Input: part model. Units: mm. Frame: model coordinates. A direction names the side the tool comes from. Coordinates: 2 decimals unless noted, no trailing zeros. Order: outer loops, then holes, each group sorted by start corner. A loop starts at its lowest first (then second) coordinate and runs counter-clockwise, first axis right, second up. Notation, with made-up numbers: (-35, 35) -> (-12, 35) arc R26 cw to (-12, 69) -> close; hole circle Ø9 at (61, 1.5). An arc over 180 degrees is marked (long way). Use one line per item in the form item = value. Start each with the question number.
1) Section query C-C on z = 0. Output: boundary loops of the cut face in (x, y) (3 decimals), then the cut area to 3 significant figures.
2) Section query B-B on y = -2.25. Output: boundary loops of the cut face in (x, z).
3) Section query D-D on z = -5.5. Output: boundary loops of the cut face in (x, y) (3 decimals), then the cut area to 3 significant figures.
4) Draft query along Y for faces 1 (the cylindrical face through (-6.97, -7.02, 0.16)), 2 (the flat face through (-3, -12.7, 3)), 3 (the cylindrical face through (-10.279, 8.343, 0.078)), 4 (the flat face through (-12.7, -3, 3)). Return one class per face: pulls with the +Y half, pulls with the -Y half, needs draft (parallel to the pull), parting line crosses it, or undercut.
5) Pin query (flat end, axial travel): pin 1 (6.5 mm diameter, centred on x = 4, z = -4.5, fed in from +Y); pin 2 (2 mm diameter, centred on x = -9, z = -7, fed in from +Y); pin 3 (11.5 mm diameter, centred on x = 0, z = 0, fed in from +Y). Return the tip coordinate at first contact, or that it passes through.
6) Ray query, line 1 along Z through (x, y) = (0, -11.2); line 2 along Y through (x, z) = (-2.25, 3); line 3 along Y through (x, z) = (-9.5, -0.25). Return the intervals inside material, ascending.
7) Access query for faces 5 (the cylindrical face through (-10.279, -3.568, -0.078)), 6 (the cylindrical face through (-3.565, -10.279, -0.157)), 7 (the flat face through (4, -7.925, 0)). Directions: +Z, -Z, +X, -X, +Y, -Y. A direction counts if a zero-diameter tool reaches every point of the face in a straight line with its end or side. Return the directions, or none.
8) Section query A-A on x = 0. Output: boundary loops of the cut face in (y, z).
from build123d import *

# Parameters (mm, degrees)
BOSS_EXTRUDE1_DEPTH      = 11.1125
BOSS_EXTRUDE1_DEPTH_BACK = 11.1125
CUT_EXTRUDE1_DEPTH       = 21.6248
CUT_EXTRUDE1_DEPTH_BACK  = 5.7752
SKETCH6_R                = 3.5687
CUT_EXTRUDE2_DEPTH       = 5.7752


with BuildPart() as part:
    # Sketch4 → Boss-Extrude1 (new body, two sides)
    with BuildSketch(Plane.XY) as boss_extrude1_sk:
        with BuildLine():
            Line((-12.7, 12.7), (-12.7, -12.7))
            Line((-12.7, -12.7), (12.7, -12.7))
            ThreePointArc((12.7, -12.7), (11.301376302, -9.323423698), (7.9248, -7.9248))
            Line((7.9248, -7.9248), (-4.7498, -7.9248))
            ThreePointArc((-4.7498, -7.9248), (-6.99486403, -6.99486403), (-7.9248, -4.7498))
            Line((-7.9248, -4.7498), (-7.9248, 7.9248))
            ThreePointArc((-7.9248, 7.9248), (-9.323423698, 11.301376302), (-12.7, 12.7))
        make_face()
    extrude(amount=BOSS_EXTRUDE1_DEPTH)
    extrude(boss_extrude1_sk.sketch, amount=-BOSS_EXTRUDE1_DEPTH_BACK)

    # Sketch5 → Cut-Extrude1 (cut, two sides)
    with BuildSketch(Plane(origin=(-7.9248, 0, 0), x_dir=(0, 0, -1), z_dir=(1, 0, 0))) as cut_extrude1_sk:
        with BuildLine():
            Line((3.5687, 4.7752), (3.5687, 0))
            ThreePointArc((3.5687, 0), (0, -3.5687), (-3.5687, 0))
            Line((-3.5687, 0), (-3.5687, 4.7752))
            ThreePointArc((-3.5687, 4.7752), (0, 8.3439), (3.5687, 4.7752))
        make_face()
    extrude(amount=CUT_EXTRUDE1_DEPTH, mode=Mode.SUBTRACT)
    extrude(cut_extrude1_sk.sketch, amount=-CUT_EXTRUDE1_DEPTH_BACK, mode=Mode.SUBTRACT)

    # Sketch6 → Cut-Extrude2 (cut, through all)
    with BuildSketch(Plane(origin=(0, -7.9248, 0), x_dir=(1, 0, 0), z_dir=(0, 1, 0))):
        Circle(SKETCH6_R)
    extrude(amount=-CUT_EXTRUDE2_DEPTH, mode=Mode.SUBTRACT)


solid = part.part
Answers below:
q1.outline = (-12.7, -12.7) -> (-3.569, -12.7) -> (-3.569, -7.925) -> (-4.75, -7.925) arc R3.175 cw to (-7.925, -4.75) -> (-7.925, -3.569) -> (-12.7, -3.569) -> close; (-12.7, 8.344) -> (-7.943, 8.344) arc R4.775 ccw to (-12.7, 12.7) -> close; (3.569, -12.7) -> (12.7, -12.7) arc R4.775 ccw to (7.925, -7.925) -> (3.569, -7.925) -> close
q1.area = 121 mm^2
q2.outline = (-12.7, -11.11) -> (-7.92, -11.11) -> (-7.92, -2.77) -> (-12.7, -2.77) -> close; (-12.7, 2.77) -> (-7.92, 2.77) -> (-7.92, 11.11) -> (-12.7, 11.11) -> close
q3.outline = (-12.7, -12.7) -> (12.7, -12.7) arc R4.775 ccw to (7.925, -7.925) -> (-4.75, -7.925) arc R3.175 cw to (-7.925, -4.75) -> (-7.925, 7.925) arc R4.775 ccw to (-12.7, 12.7) -> close
q3.area = 212 mm^2
q4.face_1 = pulls with the +Y half
q4.face_2 = pulls with the -Y half
q4.face_3 = undercut
q4.face_4 = needs draft
q5.pin_1 = -7.92
q5.pin_2 = 11.86
q5.pin_3 = -7.76
q6.line_1 = -11.11 to -3.57, 3.57 to 11.11
q6.line_2 = -12.7 to -7.92
q6.line_3 = -12.7 to -3.56, 8.34 to 11.47
q7.face_5 = +X, -X
q7.face_6 = +Y, -Y
q7.face_7 = +Z, -Z, +X, +Y
q8.outline = (-12.7, -11.11) -> (-7.92, -11.11) -> (-7.92, -3.57) -> (-12.7, -3.57) -> close; (-12.7, 3.57) -> (-7.92, 3.57) -> (-7.92, 11.11) -> (-12.7, 11.11) -> close
